Here's how the part is built. I have some questions about the finished solid (model axes, mm). Face numbers are marked on the shaded views. Coordinates: 2 decimals unless noted, no trailing zeros. Write each loop counter-clockwise with the first axis right and the second up, starting at its lowest first coordinate (ties: lowest second). Pieces come first, ordered by that corner, then holes. Notation, with made-up numbers: (71.25, 13) -> (112.25, 13) arc R19 cw to (112.25, 37) -> close; hole circle Ø9 at (17, 49.5). An arc over 180 degrees is marked (long way). Put each result on its own line as item: value. Start each with the question number.
Item 1: I want a section at B-B, the plane x = 50.8. List the corners of the cut face in (y, z) for me.
Item 2: I want a section at A-A, the plane z = -12.7. List the corners of the cut face in (x, y) for me, then the cut area to 3 significant figures.
Item 3: I want a section at C-C, the plane y = 3.25. List the corners of the cut face in (x, z) for me.
Item 4: I want a section at D-D, the plane z = -28. List the corners of the cut face in (x, y) for me.
Item 5: I need wall thicknesses on line 1 (X direction, y = 3.4, z = -12.7); line 2 (X direction, y = 2.25, z = -43); line 3 (Z direction, x = 32, y = 4). Which ranges of each line are inside material? Lowest first, please. Write a range as [from, to].
Item 6: For pin 1 (3 mm diameter, centred on x = 12.573, z = -44.196, fed in from -Y); pin 2 (6.5 mm diameter, centred on x = 89.027, z = -12.7, fed in from +Y), each with a flat end and sliding along its axis, tell me the tip position at first contact or that it passes through.
Item 7: If we mould it in two halves opening along X, with no side actions, what happens to the marked faces 1 and 2? For each: released by +X, released by -X, zero draft, split by the parting line, or undercut.
from build123d import *

# Parameters (mm, degrees)
SKETCH1_W                                            = 101.6
SKETCH1_H                                            = 50.546
BASE_DEPTH                                           = 6.35
BEARING_BLOCK_BOLT_HOLE_PATTERN_D                    = 4.2
SHAFT_CLEARANCE_HOLE_D                               = 10
PLATE_MOUNTING_WOOD_SCREW_CLEARANCE_HOLE_D           = 5.1054
PLATE_MOUNTING_WOOD_SCREW_CLEARANCE_HOLE_CSINK_D     = 9.779
PLATE_MOUNTING_WOOD_SCREW_CLEARANCE_HOLE_CSINK_ANGLE = 100


with BuildPart() as part:
    # Sketch1 → base (new body)
    with BuildSketch(Plane(origin=(0, 0, 0), x_dir=(1, 0, 0), z_dir=(0, 1, 0))):
        with Locations((50.8, 25.273)):
            Rectangle(SKETCH1_W, SKETCH1_H)
    extrude(amount=BASE_DEPTH)

    # bearing_block_bolt_hole_pattern (through all)
    with Locations(Plane(origin=(0, 6.35, 0), x_dir=(1, 0, 0), z_dir=(0, 1, 0))):
        with Locations((32.800036, 24.892), (68.799964, 24.892)):
            Hole(BEARING_BLOCK_BOLT_HOLE_PATTERN_D / 2)

    # shaft_clearance_hole (through all)
    with Locations(Plane(origin=(0, 6.35, 0), x_dir=(1, 0, 0), z_dir=(0, 1, 0))):
        with Locations((50.8, 24.892)):
            Hole(SHAFT_CLEARANCE_HOLE_D / 2)

    # plate_mounting_wood_screw_clearance_holes (through all)
    with Locations(Plane(origin=(0, 6.35, 0), x_dir=(1, 0, 0), z_dir=(0, 1, 0))):
        with Locations((12.573, 44.196), (89.027, 12.7), (12.573, 12.7), (89.027, 44.196)):
            CounterSinkHole(PLATE_MOUNTING_WOOD_SCREW_CLEARANCE_HOLE_D / 2, PLATE_MOUNTING_WOOD_SCREW_CLEARANCE_HOLE_CSINK_D / 2, counter_sink_angle=PLATE_MOUNTING_WOOD_SCREW_CLEARANCE_HOLE_CSINK_ANGLE)


solid = part.part
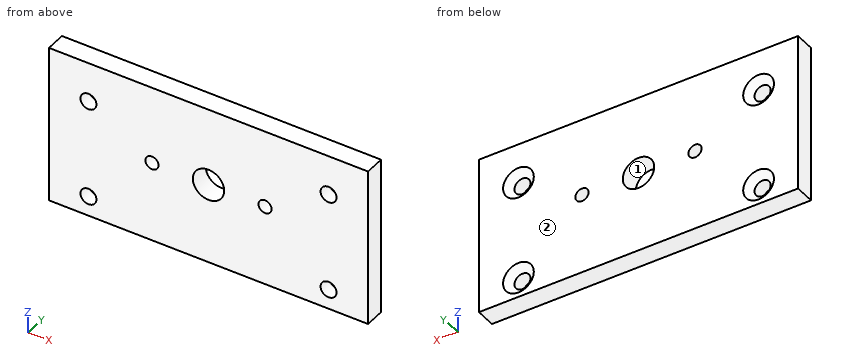
Calculated:
1. outline: (0, -50.55) -> (6.35, -50.55) -> (6.35, -29.89) -> (0, -29.89) -> close; (0, -19.89) -> (6.35, -19.89) -> (6.35, 0) -> (0, 0) -> close
2. outline: (0, 0) -> (10.02, 0) -> (10.02, 4.39) -> (7.68, 6.35) -> (0, 6.35) -> close; (15.13, 0) -> (86.47, 0) -> (86.47, 4.39) -> (84.14, 6.35) -> (17.46, 6.35) -> (15.13, 4.39) -> close; (91.58, 0) -> (101.6, 0) -> (101.6, 6.35) -> (93.92, 6.35) -> (91.58, 4.39) -> close
2. area: 571 mm2
3. outline: (0, -50.55) -> (101.6, -50.55) -> (101.6, 0) -> (0, 0) -> close; hole circle Ø5.11 at (12.57, -44.2); hole circle Ø5.11 at (12.57, -12.7); hole circle Ø4.2 at (32.8, -24.89); hole circle Ø10 at (50.8, -24.89); hole circle Ø4.2 at (68.8, -24.89); hole circle Ø5.11 at (89.03, -44.2); hole circle Ø5.11 at (89.03, -12.7)
4. outline: (0, 0) -> (46.88, 0) -> (46.88, 6.35) -> (0, 6.35) -> close; (54.72, 0) -> (101.6, 0) -> (101.6, 6.35) -> (54.72, 6.35) -> close
5. line 1: x = [0, 10.02], [15.13, 86.47], [91.58, 101.6]
5. line 2: x = [0, 10.32], [14.83, 86.77], [91.28, 101.6]
5. line 3: z = [-50.55, -26.83], [-22.95, 0]
6. pin 1: passes through
6. pin 2: stops at y = 4.97
7. face 1: undercut
7. face 2: zero draft
